Work out the finished part from the listing and answer in its coordinate system (mm). Face numbers are marked on the shaded views. Coordinates: 2 decimals unless noted, no trailing zeros. Order: outer loops, then holes, each group sorted by start corner. A loop starts at its lowest first (then second) coordinate and runs counter-clockwise, first axis right, second up. Notation, with made-up numbers: M 40.25,70.25 L 87.25,70.25 A19 cw 87.25,91.25 Z; hole C -0.5,38.25 d1. An arc over 180 degrees is marked long. Use a Markdown table: item, result.
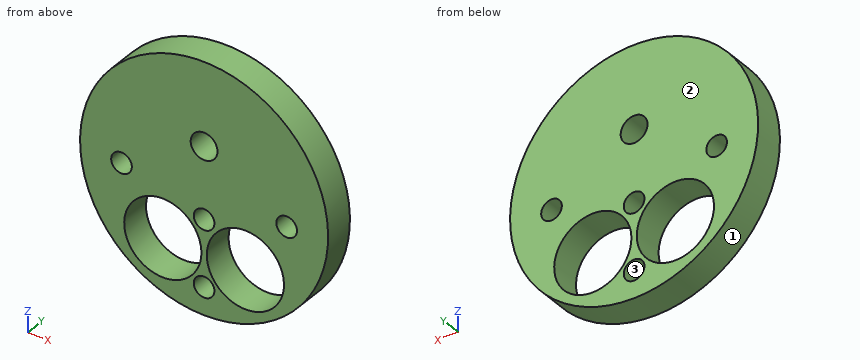
from build123d import *

# Parameters (mm, degrees)
SKETCH1_R           = 38.1508
BOSS_EXTRUDE1_DEPTH = 9.525
SKETCH19_R          = 11.8745
SKETCH19_R_2        = 3.175
CUT_EXTRUDE1_DEPTH  = 16.764
SKETCH18_R          = 3.175
CUT_EXTRUDE2_DEPTH  = 16.764
SKETCH21_R          = 4.1275
CUT_EXTRUDE3_DEPTH  = 55.787705795


with BuildPart() as part:
    # Sketch1 → Boss-Extrude1 (new body)
    with BuildSketch(Plane(origin=(0, 0, 0), x_dir=(1, 0, 0), z_dir=(0, 1, 0))):
        with Locations(Location((0, 0, 0), (0, 0, 90))):
            Circle(SKETCH1_R)
    extrude(amount=BOSS_EXTRUDE1_DEPTH)

    # Sketch19 → Cut-Extrude1 (cut)
    with BuildSketch(Plane(origin=(0, 9.525, 0), x_dir=(1, 0, 0), z_dir=(0, 1, 0))):
        with Locations(Location((-12.7, 19.685, 0), (0, 0, 270))):
            Circle(SKETCH19_R)
        with Locations(Location((12.7, 19.685, 0), (0, 0, 270))):
            Circle(SKETCH19_R)
        with Locations(Location((0, 29.654011512, 0), (0, 0, 270))):
            Circle(SKETCH19_R_2)
        with Locations(Location((0, 9.334011512, 0), (0, 0, 270))):
            Circle(SKETCH19_R_2)
    extrude(amount=-CUT_EXTRUDE1_DEPTH, mode=Mode.SUBTRACT)

    # Sketch18 → Cut-Extrude2 (cut)
    with BuildSketch(Plane(origin=(0, 9.525, 0), x_dir=(1, 0, 0), z_dir=(0, 1, 0))):
        with Locations(Location((25.4, 1.905, 0), (0, 0, 270))):
            Circle(SKETCH18_R)
        with Locations(Location((-25.4, 1.905, 0), (0, 0, 270))):
            Circle(SKETCH18_R)
    extrude(amount=-CUT_EXTRUDE2_DEPTH, mode=Mode.SUBTRACT)

    # Sketch21 → Cut-Extrude3 (cut, through all)
    with BuildSketch(Plane(origin=(0, 9.525, 0), x_dir=(1, 0, 0), z_dir=(0, 1, 0))):
        with Locations(Location((0, -12.7, 0), (0, 0, 270))):
            Circle(SKETCH21_R)
    extrude(amount=-CUT_EXTRUDE3_DEPTH, mode=Mode.SUBTRACT)


solid = part.part
(1) A cutting plane is placed at B-B (y = 4). Give the number of separate pieces and of enclosed holes in the cut face, then the cut area to 3 significant figures.
Conclusion:
| item | result |
|---|---|
| separate pieces | 1 |
| enclosed holes | 7 |
| area | 3,510 mm2 |
(2) Given P1, Ø19, axis at x = -12.7, z = -19.685, coming from the -Y side; P2, Ø1, axis at x = -5, y = 4, coming from the -Z side; P3, Ø5, axis at x = -25.5, y = 3, coming from the +Z side; P4, Ø4, axis at y = 3, z = 0.5, coming from the +X side, each flat-ended and moving along its own axis, determine where each tip first touches the part or whether it passes through.
Conclusion:
| item | result |
|---|---|
| P1 | through |
| P2 | z = -37.88 |
| P3 | z = 30.44 |
| P4 | x = 38.15 |
(3) A cutting plane is placed at A-A (z = 0). Determine the outline of the cut face in (x, y) (3 decimals), then the cut area to 3 significant figures.
Conclusion:
| item | result |
|---|---|
| outline | M -38.151,0 L -27.94,0 L -27.94,9.525 L -38.151,9.525 Z; M -22.86,0 L 22.86,0 L 22.86,9.525 L -22.86,9.525 Z; M 27.94,0 L 38.151,0 L 38.151,9.525 L 27.94,9.525 Z |
| area | 630 mm2 |
(4) Determine the mould class of the marked faces 1, 2 and 3 for opening direction X: pulls with the +X half, pulls with the -X half, needs draft (parallel to the pull), parting line crosses it, or undercut.
Conclusion:
| item | result |
|---|---|
| face 1 | parting line crosses it |
| face 2 | needs draft |
| face 3 | undercut |
(5) Straight lines are drawn through the part: L1, parallel to Z at x = 23, y = 4.75; L2, parallel to X at y = 6.5, z = -17.5; L3, parallel to Z at x = -31, y = 3. For each, find the intervals that lie inside material, in ascending order.
Conclusion:
| item | result |
|---|---|
| L1 | -30.44 to -25.59, -13.78 to -3.98, 0.17 to 30.44 |
| L2 | -33.9 to -24.37, -1.03 to 1.03, 24.37 to 33.9 |
| L3 | -22.24 to 22.24 |
(6) A cutting plane is placed at C-C (x = 12.7). Determine the outline of the cut face in (y, z) (1 decimal), then the cut area to 3 significant figures.
Conclusion:
| item | result |
|---|---|
| outline | M 0,-36 L 9.5,-36 L 9.5,-31.6 L 0,-31.6 Z; M 0,-7.8 L 9.5,-7.8 L 9.5,36 L 0,36 Z |
| area | 459 mm2 |
(7) A cutting plane is placed at D-D (z = -11.5). Determine the outline of the cut face in (x, y) (3 decimals), then the cut area to 3 significant figures.
Conclusion:
| item | result |
|---|---|
| outline | M -36.376,0 L -21.303,0 L -21.303,9.525 L -36.376,9.525 Z; M -4.097,0 L -2.321,0 L -2.321,9.525 L -4.097,9.525 Z; M 2.321,0 L 4.097,0 L 4.097,9.525 L 2.321,9.525 Z; M 21.303,0 L 36.376,0 L 36.376,9.525 L 21.303,9.525 Z |
| area | 321 mm2 |
